from build123d import *

# Parameters (mm, degrees)
SKETCH2_W            = 5
SKETCH2_H            = 5
PACKAGE_DEPTH        = 1.5
DRAFT1_START         = -2.5
DRAFT1_DEPTH         = 5
DRAFT1_START_2       = -3
DRAFT1_2_DEPTH       = 6
DRAFT2_START         = -2.5
DRAFT2_DEPTH         = 5
DRAFT2_START_2       = -3
DRAFT2_2_DEPTH       = 6
CHAMFER1_SIZE        = 0.25
CHAMFER1_SIZE2       = 0.275015717
LEADS_DEPTH          = 0.2
FILLET1_R            = 0.25
FILLET2_R            = 0.125
FILLET1_OF_MIRROR1_R = 0.25
FILLET2_OF_MIRROR1_R = 0.125
LPATTERN1_START      = -0.835
LPATTERN1_DEPTH      = 0.4
LPATTERN1_START_2    = 0.435
LPATTERN1_2_DEPTH    = 0.4
LPATTERN1_START_3    = 1.705
LPATTERN1_3_DEPTH    = 0.4
SKETCH4_R            = 0.225
MARKER_DEPTH         = 0.1


with BuildPart() as part:
    # Sketch2 → Package (new body)
    with BuildSketch(Plane(origin=(0, 0.25, 0), x_dir=(-1, 0, 0), z_dir=(0, 1, 0))):
        Rectangle(SKETCH2_W, SKETCH2_H)
    extrude(amount=PACKAGE_DEPTH)

    # Draft1: read off the stored shape, not the designer's step
    # Draft1 outline → Draft1 (cut)
    with BuildSketch(Plane.YZ.offset(DRAFT1_START)):
        Polygon((1.75, -2.5), (1.75, -2.434383502), (1, -2.5), align=None)
        Polygon((1, 2.5), (1.75, 2.434383502), (1.75, 2.5), align=None)
    extrude(amount=DRAFT1_DEPTH, mode=Mode.SUBTRACT)

    # Draft1 2 outline → Draft1 2 (cut)
    with BuildSketch(Plane.XY.offset(DRAFT1_START_2)):
        Polygon((-2.5, 1), (-2.434383502, 1.75), (-2.5, 1.75), align=None)
        Polygon((2.434383502, 1.75), (2.5, 1), (2.5, 1.75), align=None)
    extrude(amount=DRAFT1_2_DEPTH, mode=Mode.SUBTRACT)

    # Draft2: read off the stored shape, not the designer's step
    # Draft2 outline → Draft2 (cut)
    with BuildSketch(Plane.XY.offset(DRAFT2_START)):
        Polygon((2.5, 0.75), (2.456255668, 0.25), (2.5, 0.25), align=None)
        Polygon((-2.456255668, 0.25), (-2.5, 0.75), (-2.5, 0.25), align=None)
    extrude(amount=DRAFT2_DEPTH, mode=Mode.SUBTRACT)

    # Draft2 2 outline → Draft2 2 (cut)
    with BuildSketch(Plane.YZ.offset(DRAFT2_START_2)):
        Polygon((0.75, -2.5), (0.25, -2.456255668), (0.25, -2.5), align=None)
        Polygon((0.25, 2.456255668), (0.75, 2.5), (0.25, 2.5), align=None)
    extrude(amount=DRAFT2_2_DEPTH, mode=Mode.SUBTRACT)

    # Chamfer1
    chamfer1_edges = [part.edges().sort_by_distance(p)[0] for p in [
        (0, 1.75, 2.434383502),
    ]]
    chamfer1_side = [part.faces().sort_by_distance(p)[0] for p in [
        (0, 1.373337774, 2.467337177),
    ]]
    chamfer(chamfer1_edges, length=CHAMFER1_SIZE, length2=CHAMFER1_SIZE2, reference=chamfer1_side[0])

    # Sketch3 → Leads (add, symmetric)
    with BuildSketch(Plane.ZY.offset(1.905)):
        Polygon((-2.5, 1), (-2.5, 0.75), (3, 0.75), (3, 0), (3.6, 0), (3.6, 0.25), (3.25, 0.25), (3.25, 1), align=None)
    leads = extrude(amount=LEADS_DEPTH, both=True)

    # Fillet1
    fillet1_edges = [part.edges().sort_by_distance(p)[0] for p in [
        (-1.905, 1, 3.25),
        (-1.905, 0, 3),
    ]]
    fillet(fillet1_edges, radius=FILLET1_R)

    # Fillet2
    fillet2_edges = [part.edges().sort_by_distance(p)[0] for p in [
        (-1.905, 0.75, 3),
        (-1.905, 0.25, 3.25),
    ]]
    fillet(fillet2_edges, radius=FILLET2_R)

    # Mirror1: Leads across plane
    add(leads.mirror(Plane.XY))

    # Fillet1 of Mirror1
    fillet1_of_mirror1_edges = [part.edges().sort_by_distance(p)[0] for p in [
        (-1.905, 1, -3.25),
        (-1.905, 0, -3),
    ]]
    fillet(fillet1_of_mirror1_edges, radius=FILLET1_OF_MIRROR1_R)

    # Fillet2 of Mirror1
    fillet2_of_mirror1_edges = [part.edges().sort_by_distance(p)[0] for p in [
        (-1.905, 0.75, -3),
        (-1.905, 0.25, -3.25),
    ]]
    fillet(fillet2_of_mirror1_edges, radius=FILLET2_OF_MIRROR1_R)

    # LPattern1: read off the stored shape, not the designer's step
    # LPattern1 outline → LPattern1 (add)
    with BuildSketch(Plane.YZ.offset(LPATTERN1_START)):
        with BuildLine():
            Line((1, 2.5), (1, 3))
            ThreePointArc((1, 3), (0.926776695, 3.176776695), (0.75, 3.25))
            Line((0.75, 3.25), (0.375, 3.25))
            ThreePointArc((0.375, 3.25), (0.286611652, 3.286611652), (0.25, 3.375))
            Line((0.25, 3.375), (0.25, 3.6))
            Line((0.25, 3.6), (0, 3.6))
            Line((0, 3.6), (0, 3.25))
            ThreePointArc((0, 3.25), (0.073223305, 3.073223305), (0.25, 3))
            Line((0.25, 3), (0.625, 3))
            ThreePointArc((0.625, 3), (0.713388348, 2.963388348), (0.75, 2.875))
            Line((0.75, 2.875), (0.75, 2.5))
            Line((0.75, 2.5), (1, 2.5))
        make_face()
        with BuildLine():
            ThreePointArc((0.75, -3.25), (0.926776695, -3.176776695), (1, -3))
            Line((1, -3), (1, -2.5))
            Line((1, -2.5), (0.75, -2.5))
            Line((0.75, -2.5), (0.75, -2.875))
            ThreePointArc((0.75, -2.875), (0.713388348, -2.963388348), (0.625, -3))
            Line((0.625, -3), (0.25, -3))
            ThreePointArc((0.25, -3), (0.073223305, -3.073223305), (0, -3.25))
            Line((0, -3.25), (0, -3.6))
            Line((0, -3.6), (0.25, -3.6))
            Line((0.25, -3.6), (0.25, -3.375))
            ThreePointArc((0.25, -3.375), (0.286611652, -3.286611652), (0.375, -3.25))
            Line((0.375, -3.25), (0.75, -3.25))
        make_face()
    extrude(amount=LPATTERN1_DEPTH)

    # LPattern1 2 outline → LPattern1 2 (add)
    with BuildSketch(Plane.YZ.offset(LPATTERN1_START_2)):
        with BuildLine():
            Line((1, 2.5), (1, 3))
            ThreePointArc((1, 3), (0.926776695, 3.176776695), (0.75, 3.25))
            Line((0.75, 3.25), (0.375, 3.25))
            ThreePointArc((0.375, 3.25), (0.286611652, 3.286611652), (0.25, 3.375))
            Line((0.25, 3.375), (0.25, 3.6))
            Line((0.25, 3.6), (0, 3.6))
            Line((0, 3.6), (0, 3.25))
            ThreePointArc((0, 3.25), (0.073223305, 3.073223305), (0.25, 3))
            Line((0.25, 3), (0.625, 3))
            ThreePointArc((0.625, 3), (0.713388348, 2.963388348), (0.75, 2.875))
            Line((0.75, 2.875), (0.75, 2.5))
            Line((0.75, 2.5), (1, 2.5))
        make_face()
        with BuildLine():
            ThreePointArc((0.75, -3.25), (0.926776695, -3.176776695), (1, -3))
            Line((1, -3), (1, -2.5))
            Line((1, -2.5), (0.75, -2.5))
            Line((0.75, -2.5), (0.75, -2.875))
            ThreePointArc((0.75, -2.875), (0.713388348, -2.963388348), (0.625, -3))
            Line((0.625, -3), (0.25, -3))
            ThreePointArc((0.25, -3), (0.073223305, -3.073223305), (0, -3.25))
            Line((0, -3.25), (0, -3.6))
            Line((0, -3.6), (0.25, -3.6))
            Line((0.25, -3.6), (0.25, -3.375))
            ThreePointArc((0.25, -3.375), (0.286611652, -3.286611652), (0.375, -3.25))
            Line((0.375, -3.25), (0.75, -3.25))
        make_face()
    extrude(amount=LPATTERN1_2_DEPTH)

    # LPattern1 3 outline → LPattern1 3 (add)
    with BuildSketch(Plane.YZ.offset(LPATTERN1_START_3)):
        with BuildLine():
            Line((1, 2.5), (1, 3))
            ThreePointArc((1, 3), (0.926776695, 3.176776695), (0.75, 3.25))
            Line((0.75, 3.25), (0.375, 3.25))
            ThreePointArc((0.375, 3.25), (0.286611652, 3.286611652), (0.25, 3.375))
            Line((0.25, 3.375), (0.25, 3.6))
            Line((0.25, 3.6), (0, 3.6))
            Line((0, 3.6), (0, 3.25))
            ThreePointArc((0, 3.25), (0.073223305, 3.073223305), (0.25, 3))
            Line((0.25, 3), (0.625, 3))
            ThreePointArc((0.625, 3), (0.713388348, 2.963388348), (0.75, 2.875))
            Line((0.75, 2.875), (0.75, 2.5))
            Line((0.75, 2.5), (1, 2.5))
        make_face()
        with BuildLine():
            ThreePointArc((0.75, -3.25), (0.926776695, -3.176776695), (1, -3))
            Line((1, -3), (1, -2.5))
            Line((1, -2.5), (0.75, -2.5))
            Line((0.75, -2.5), (0.75, -2.875))
            ThreePointArc((0.75, -2.875), (0.713388348, -2.963388348), (0.625, -3))
            Line((0.625, -3), (0.25, -3))
            ThreePointArc((0.25, -3), (0.073223305, -3.073223305), (0, -3.25))
            Line((0, -3.25), (0, -3.6))
            Line((0, -3.6), (0.25, -3.6))
            Line((0.25, -3.6), (0.25, -3.375))
            ThreePointArc((0.25, -3.375), (0.286611652, -3.286611652), (0.375, -3.25))
            Line((0.375, -3.25), (0.75, -3.25))
        make_face()
    extrude(amount=LPATTERN1_3_DEPTH)

    # Sketch4 → Marker (cut)
    with BuildSketch(Plane(origin=(0, 1.75, 0), x_dir=(1, 0, 0), z_dir=(0, 1, 0))):
        with Locations(Location((-1.905, -1.2, 0), (0, 0, 270))):
            Circle(SKETCH4_R)
    extrude(amount=-MARKER_DEPTH, mode=Mode.SUBTRACT)


solid = part.part
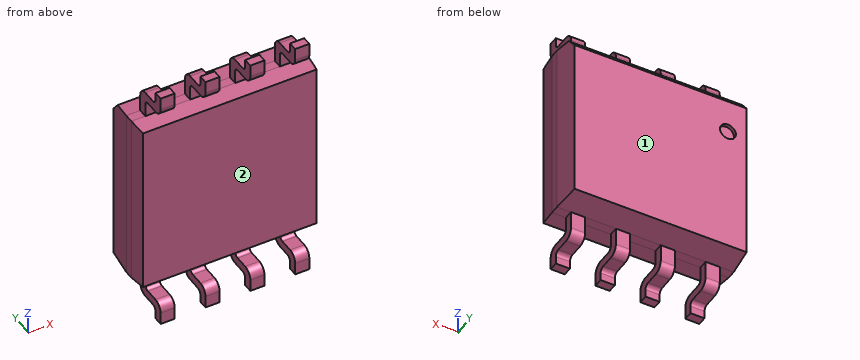
Model file for the job. Use its own axes, mm. Face numbers are marked on the shaded views. Give positions to 0.01 mm unless a question says otherwise; leave off trailing zeros. Loops run counter-clockwise (first coordinate to the right, second up) from the corner with the lowest first, then second, coordinate; pieces in that order, holes last. Notation, with made-up numbers: (40, 88) -> (86, 88) arc R29 cw to (86, 118) -> close; hole circle Ø9 at (69, 13.5). An arc over 180 degrees is marked (long way). Use a Markdown table: item, result. Add a question column.
(1) Drop a flat-ended pin along its axis: pin 1 Ø0.8 at (y, z) = (0.5, -3) entering from -X (3 decimals). Give the stop position or say it passes through.
(2) Slice it at B-B on z = 1.2. List the corners of the cut face in (x, y).
(3) Slice it at D-D on z = 0.25. List the corners of the cut face in (x, y), and give its area (3 significant figures).
(4) Slice it at C-C on y = 1.35. List the corners of the cut face in (x, z), and give its area (3 significant figures).
(5) Mould opens along Z. For the marked faces 1 and 2 say: +Z half, -Z half, draft (parallel to the pull), parting line (faces both ways), or undercut.
(6) Wall check: line 1 along Z through (x, y) = (0.05, 0.75); line 2 along X through (y, z) = (1.7, 1.2); line 3 along Y through (x, z) = (-0.55, -1). Give the ranges that are in metal, low to high.
(7) Slice it at A-A on x = -0.2. List the corners of the cut face in (y, z), and give its area (3 significant figures).
Filled sheet:
| question | item | result |
|---|---|---|
| 1 | pin 1 | x = -2.105 |
| 2 | outline | (-2.5, 0.75) -> (-2.46, 0.25) -> (2.46, 0.25) -> (2.5, 0.75) -> (2.5, 1) -> (2.43, 1.75) -> (-1.68, 1.75) -> (-1.68, 1.65) -> (-2.13, 1.65) -> (-2.13, 1.75) -> (-2.43, 1.75) -> (-2.5, 1) -> close |
| 3 | outline | (-2.5, 0.75) -> (-2.46, 0.25) -> (2.46, 0.25) -> (2.5, 0.75) -> (2.5, 1) -> (2.43, 1.75) -> (-2.43, 1.75) -> (-2.5, 1) -> close |
| 3 | area | 7.43 mm2 |
| 4 | outline | (-2.47, -2.47) -> (2.47, -2.47) -> (2.47, 2.47) -> (-2.47, 2.47) -> close |
| 4 | area | 24.4 mm2 |
| 5 | face 1 | draft |
| 5 | face 2 | undercut |
| 6 | line 1 | -2.5 to 2.5 |
| 6 | line 2 | -2.44 to -2.13, -1.68 to 2.44 |
| 6 | line 3 | 0.25 to 1.75 |
| 7 | outline | (0.25, -2.46) -> (0.75, -2.5) -> (1, -2.5) -> (1.75, -2.43) -> (1.75, 2.16) -> (1.5, 2.46) -> (1, 2.5) -> (0.75, 2.5) -> (0.25, 2.46) -> close |
| 7 | area | 7.39 mm2 |
